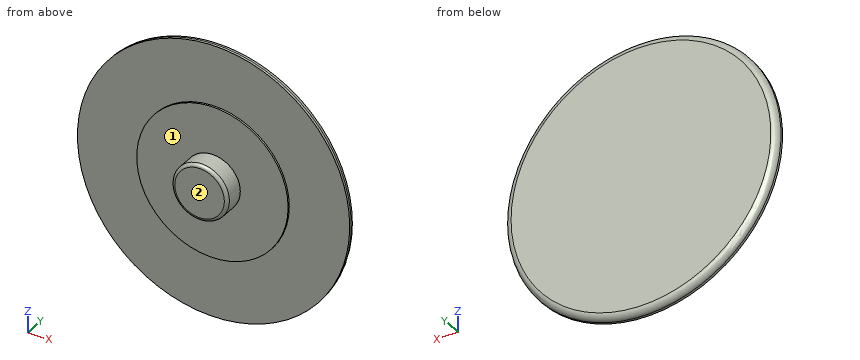
from build123d import *

# Parameters (mm, degrees)
F2_R     = 4.478894
F3_DEPTH = 5
F1_R     = 12.160504
F4_DEPTH = 1.7
F0_R     = 21.8645
F5_DEPTH = 1.4
F6_R     = 1
F7_R     = 0.5


with BuildPart() as f3:
    # F2 (on Front) → F3 (new body)
    with BuildSketch(Plane.XZ):
        Circle(F2_R)
    extrude(amount=F3_DEPTH)

    # F1 (on Front) → F4 (join)
    with BuildSketch(Plane.XZ):
        Circle(F1_R)
    extrude(amount=F4_DEPTH)

    # F0 (on Front) → F5 (join)
    with BuildSketch(Plane.XZ):
        Circle(F0_R)
    extrude(amount=F5_DEPTH)

    # F6
    f6_edges = [f3.edges().sort_by_distance(p)[0] for p in [
        (-21.8645, 0, 0),
    ]]
    fillet(f6_edges, radius=F6_R)

    # F7
    f7_edges = [f3.edges().sort_by_distance(p)[0] for p in [
        (-4.478894, -5, 0),
    ]]
    fillet(f7_edges, radius=F7_R)


solid = f3.part
Verification items for the finished model (mm, model axes). Face numbers are marked on the shaded views. A direction names the side the tool comes from. Give positions to 0.01 mm unless a question says otherwise; leave off trailing zeros. Loops run counter-clockwise (first coordinate to the right, second up) from the corner with the lowest first, then second, coordinate; pieces in that order, holes last.
1) Sectioned sample at B-B, the plane z = 0. Enter the section's corners in (x, y).
2) Thickness scan on line 1 along Y through (x, z) = (11, -8.5); line 2 along Y through (x, z) = (-4.5, 1); line 3 along X through (y, z) = (-1.6, 0.5). Record the ranges inside material, lowest first.
3) Sectioned sample at A-A, the plane x = 0. Enter the section's corners in (y, z).
4) Set-up check for the marked faces 1 and 2: record each of +Z, -Z, +X, -X, +Y, -Y from which the full face is reachable in a straight line by a thin tool's end or side.
5) Depth check by flat-ended pin: pin 1 Ø7.5 at (x, z) = (-3.5, 5.5) entering from -Y; pin 2 Ø10 at (x, z) = (9.5, 6) entering from -Y; pin 3 Ø3 at (x, z) = (13.5, -9.5) entering from -Y; pin 4 Ø3 at (y, z) = (-1.5, -12.5) entering from +X. Enter the tip coordinate at first touch or a pass-through.
Answers:
1. outline: (-21.86, -1.4) - (-12.16, -1.4) - (-12.16, -1.7) - (-4.48, -1.7) - (-4.48, -4.5) arc R0.5 ccw to (-3.98, -5) - (3.98, -5) arc R0.5 ccw to (4.48, -4.5) - (4.48, -1.7) - (12.16, -1.7) - (12.16, -1.4) - (21.86, -1.4) - (21.86, -1) arc R1 ccw to (20.86, 0) - (-20.86, 0) arc R1 ccw to (-21.86, -1) - close
2. line 1: y = -1.4 to 0
2. line 2: y = -1.7 to 0
2. line 3: x = -12.15 to 12.15
3. outline: (-5, -3.98) arc R0.5 ccw to (-4.5, -4.48) - (-1.7, -4.48) - (-1.7, -12.16) - (-1.4, -12.16) - (-1.4, -21.86) - (-1, -21.86) arc R1 ccw to (0, -20.86) - (0, 20.86) arc R1 ccw to (-1, 21.86) - (-1.4, 21.86) - (-1.4, 12.16) - (-1.7, 12.16) - (-1.7, 4.48) - (-4.5, 4.48) arc R0.5 ccw to (-5, 3.98) - close
4. face 1: -Y
4. face 2: +Z, -Z, +X, -X, -Y
5. pin 1: stops at y = -5
5. pin 2: stops at y = -1.7
5. pin 3: stops at y = -1.4
5. pin 4: stops at x = 18.89
